Can you work these out from the model? Positions are in its coordinate system, mm. A direction names the side the tool comes from. Coordinates: 2 decimals unless noted, no trailing zeros. Order: outer loops, then holes, each group sorted by start corner. A loop starts at its lowest first (then second) coordinate and runs counter-clockwise, first axis right, second up. Notation, with made-up numbers: M -38,-0.75 L -26,-0.75 A28 cw -26,21.25 Z; hole C 12.5,19.25 d10. An arc over 180 degrees is marked long. Answer as CSV lines item,"result". Start each with the question number.
1. If we section it at A-A (y = 1.25): List the corners of the cut face in (x, z) for me, plus the area to 3 significant figures.
2. If we section it at B-B (z = -2.3): List the corners of the cut face in (x, y) for me, plus the area to 3 significant figures.
3. If we mould it in two halves opening along X, with no side actions, what happens to faces 1 (the face through (1.5, 8, -3.2)), 2 (the face through (7.465, 6.902, -29.926)), 3 (the face through (8, 5, -46))? For each: released by +X, released by -X, zero draft, split by the parting line, or undercut.
4. Will these pins go through, and if not, where does the flat tip stop? pin 1 (5 mm diameter, centred on y = 7.28, z = -2.3, fed in from -X); pin 2 (3 mm diameter, centred on x = 3, y = 1.5, fed in from -Z); pin 3 (1 mm diameter, centred on y = 7, z = -7.5, fed in from +X).
5. If we section it at C-C (y = 7.28): List the corners of the cut face in (x, z) for me, plus the area to 3 significant figures.
6. On a 3-axis mill with a long thin cutter (end or side, diameter ignored), from which of +Z, -Z, +X, -X, +Y, -Y can I reach the whole of each face in a straight line? I mean faces 4 (the face through (5, 7, -43)), 5 (the face through (3, 5, -5)), 6 (the face through (5, 7, -14)), 7 (the face through (0.74, 7.38, -5.15)). Say none if no direction works.
7. I need wall thicknesses on line 1 along Y through (x, z) = (1.1, -2.3); line 2 along X through (y, z) = (2, -46); line 3 along X through (y, z) = (0.5, -40.5). Which ranges of each line are inside material? Lowest first, please. Write a range as from..to.
8. If we section it at D-D (x = 2): List the corners of the cut face in (y, z) for me, plus the area to 3 significant figures.
```python
from build123d import *

# Parameters (mm, degrees)
SALIENTE_EXTRUIR1_DEPTH = 14
CROQUIS3_R              = 1
CORTAR_EXTRUIR1_DEPTH   = 5
CROQUIS5_R              = 2.85
CORTAR_EXTRUIR2_DEPTH   = 1.5
CROQUIS6_R              = 0.94
CORTAR_EXTRUIR3_DEPTH   = 54.279827327


with BuildPart() as part:
    # Croquis1 → Saliente-Extruir1 (new body)
    with BuildSketch(Plane(origin=(0, 0, 0), x_dir=(1, 0, 0), z_dir=(0, 1, 0))):
        Polygon((0, 0), (5, 0), (5, 28.2), (10, 31.7), (10, 50.7), (5, 50.7), (5, 35.2), (0, 31.7), align=None)
    extrude(amount=SALIENTE_EXTRUIR1_DEPTH)

    # Croquis3 → Cortar-Extruir1 (cut)
    with BuildSketch(Plane.XZ):
        with Locations(Location((2.5, -4.7, 0), (0, 0, 270))):
            Circle(CROQUIS3_R)
        with Locations(Location((7.5, -46, 0), (0, 0, 270))):
            Circle(CROQUIS3_R)
    extrude(amount=-CORTAR_EXTRUIR1_DEPTH, mode=Mode.SUBTRACT)

    # Croquis5 → Cortar-Extruir2 (cut)
    with BuildSketch(Plane.ZY):
        with Locations((-2.3, 7.28)):
            Circle(CROQUIS5_R)
    extrude(amount=-CORTAR_EXTRUIR2_DEPTH, mode=Mode.SUBTRACT)

    # Croquis6 → Cortar-Extruir3 (cut, through all)
    with BuildSketch(Plane.ZY.offset(-1.5)):
        with Locations((-2.3, 7.28)):
            Circle(CROQUIS6_R)
    extrude(amount=-CORTAR_EXTRUIR3_DEPTH, mode=Mode.SUBTRACT)


solid = part.part
```
Solved:
1,outline,"M 0,-31.7 L 5,-35.2 L 5,-50.7 L 10,-50.7 L 10,-31.7 L 5,-28.2 L 5,0 L 0,0 Z; hole C 2.5,-4.7 d2; hole C 7.5,-46 d2"
1,area,"265 mm²"
2,outline,"M 0,0 L 5,0 L 5,6.34 L 1.5,6.34 L 1.5,4.43 L 0,4.43 Z; M 0,10.13 L 1.5,10.13 L 1.5,8.22 L 5,8.22 L 5,14 L 0,14 Z"
2,area,"54.9 mm²"
3,face 1,"released by -X"
3,face 2,"released by +X"
3,face 3,"undercut"
4,pin 1,"x = 1.5"
4,pin 2,"z = -34.85"
4,pin 3,"x = 5"
5,outline,"M 0,-31.7 L 5,-35.2 L 5,-50.7 L 10,-50.7 L 10,-31.7 L 5,-28.2 L 5,-3.24 L 1.5,-3.24 L 1.5,-5.15 L 0,-5.15 Z; M 1.5,-1.36 L 5,-1.36 L 5,0 L 1.5,0 Z"
5,area,"257 mm²"
6,face 4,"-Z, -X, +Y, -Y"
6,face 5,"-Y"
6,face 6,"+Z, +X, +Y, -Y"
6,face 7,"-X"
7,line 1,"0..4.43, 10.13..14"
7,line 2,"5..6.5, 8.5..10"
7,line 3,"5..10"
8,outline,"M 0,-33.1 L 14,-33.1 L 14,0 L 0,0 L 0,-3.83 L 5,-3.83 L 5,-5.57 L 0,-5.57 Z; hole C 7.28,-2.3 d1.88"
8,area,"452 mm²"
